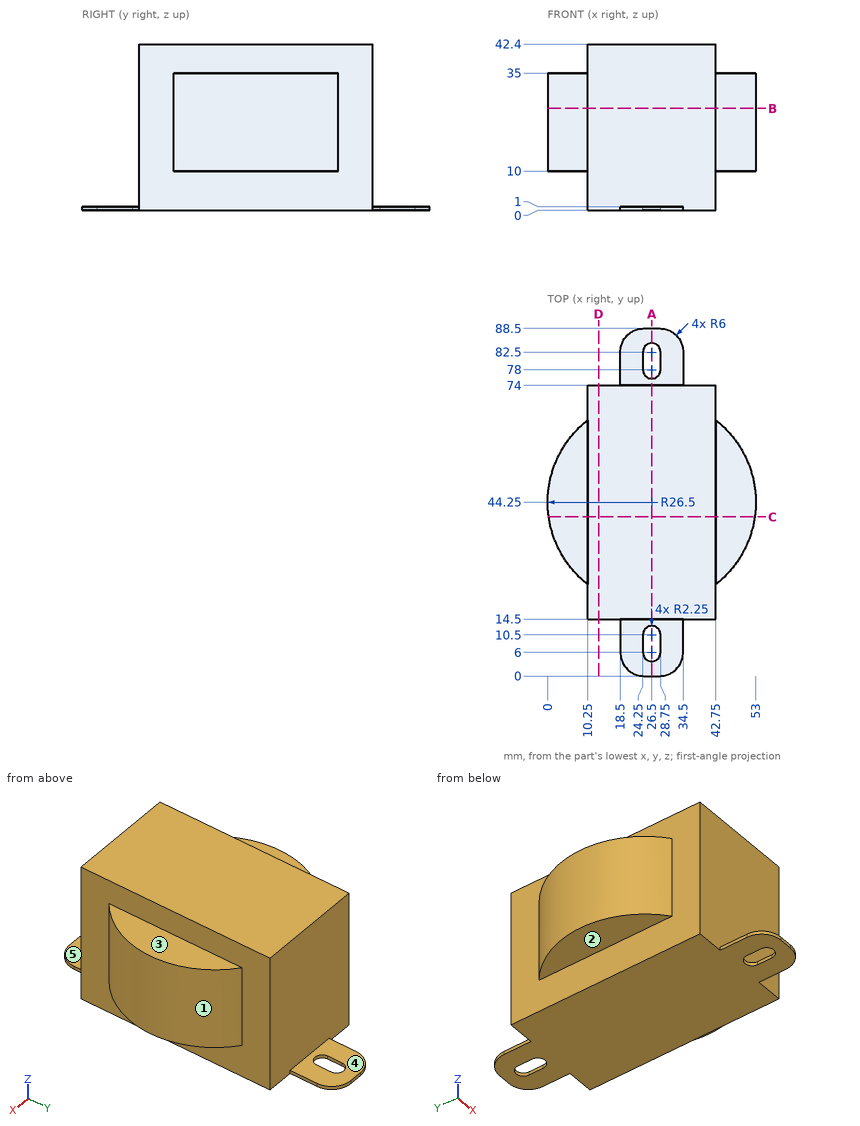
Verification items for this drawing (mm, ordinates from the low corner). A direction names the side the tool comes from. Coordinates: 2 decimals unless noted, no trailing zeros. Loops run counter-clockwise (first coordinate to the right, second up) from the corner with the lowest first, then second, coordinate; pieces in that order, holes last. Notation, with made-up numbers: (82, 29.25) -> (90, 29.25) arc R16 cw to (90, 36.25) -> close; hole circle Ø7 at (28, 43.25). An arc over 180 degrees is marked (long way). Answer in a Markdown table with one row per item. Add a question column.
1. Depth check by flat-ended pin: P1, Ø1, axis at x = 32.5, z = 8, coming from the +Y side; P2, Ø2, axis at y = 16.5, z = 30.5, coming from the -X side; P3, Ø1.1, axis at y = 12.5, z = 0.5, coming from the +X side; P4, Ø1, axis at x = 9.5, z = 9, coming from the +Y side. Enter the tip coordinate at first touch or a pass-through.
2. Section check A-A, the plane x = 26.5. Enter the section's corners in (y, z), then the cut area to 3 significant figures.
3. Section check D-D, the plane x = 13. Enter the section's corners in (y, z), then the cut area to 3 significant figures.
4. Access from +Z, -Z, +X, -X, +Y, -Y to the whole of each face (thin tool, end or side, straight path). Record for the marked faces 1, 2, 3, 4 and 5.
5. Section check B-B, the plane z = 26. Enter the section's corners in (x, y).
6. Material ranges on probe 1 along Y at (x, z) = (18.5, 20.5); probe 2 along X at (y, z) = (33, 9); probe 3 along X at (y, z) = (43.5, 34.5), recorded low to high. Write a range as [from, to].
7. Section check C-C, the plane y = 40.5. Enter the section's corners in (x, z), then the cut area to 3 significant figures.
Derived:
| question | item | result |
|---|---|---|
| 1 | P1 | stops at y = 74 |
| 1 | P2 | stops at x = 10.25 |
| 1 | P3 | stops at x = 34.5 |
| 1 | P4 | passes through |
| 2 | outline | (0, 0) -> (3.75, 0) -> (3.75, 1) -> (0, 1) -> close; (12.75, 0) -> (75.75, 0) -> (75.75, 1) -> (74, 1) -> (74, 42.4) -> (14.5, 42.4) -> (14.5, 1) -> (12.75, 1) -> close; (84.75, 0) -> (88.5, 0) -> (88.5, 1) -> (84.75, 1) -> close |
| 2 | area | 2,530 mm² |
| 3 | outline | (14.5, 0) -> (74, 0) -> (74, 42.4) -> (14.5, 42.4) -> close |
| 3 | area | 2,520 mm² |
| 4 | face 1 | +Z, -Z, +X |
| 4 | face 2 | -Z, -X, +Y, -Y |
| 4 | face 3 | +Z, +X, +Y, -Y |
| 4 | face 4 | +Z, +X, -X, +Y |
| 4 | face 5 | +Z, +X, -X, -Y |
| 5 | outline | (10.25, 14.5) -> (42.75, 14.5) -> (42.75, 23.32) arc R26.5 ccw to (42.75, 65.18) -> (42.75, 74) -> (10.25, 74) -> (10.25, 65.18) arc R26.5 ccw to (10.25, 23.32) -> close |
| 6 | probe 1 | y = [14.5, 74] |
| 6 | probe 2 | x = [10.25, 42.75] |
| 6 | probe 3 | x = [0.01, 52.99] |
| 7 | outline | (0.27, 10) -> (10.25, 10) -> (10.25, 0) -> (42.75, 0) -> (42.75, 10) -> (52.73, 10) -> (52.73, 35) -> (42.75, 35) -> (42.75, 42.4) -> (10.25, 42.4) -> (10.25, 35) -> (0.27, 35) -> close |
| 7 | area | 1,880 mm² |
